Answer from the drawing. Dimensions are ordinates in mm from the lowest x, y and z of the part. A direction names the side the tool comes from. Coordinates: 2 decimals unless noted, no trailing zeros. Order: outer loops, then holes, each group sorted by start corner. A loop starts at its lowest first (then second) coordinate and runs counter-clockwise, first axis right, second up. Notation, with made-up numbers: (-11.75, 27) -> (41.25, 27) arc R24 ccw to (41.25, 47) -> close; hole circle Ø6 at (-15.75, 37.5). An arc over 180 degrees is marked (long way). Answer as a JSON object with one key per item and string values. Group by question number.
1) Section A-A on z = 14.5 is taken. Determine the outline of the cut face in (x, y), and give its area (3 significant figures).
2) Section B-B on x = 20 is taken. Determine the outline of the cut face in (y, z), and give its area (3 significant figures).
3) Determine the mould class of the marked faces 1, 2 and 3 for opening direction X: released by +X, released by -X, zero draft, split by the parting line, or undercut.
4) Section C-C on y = 15 is taken. Determine the outline of the cut face in (x, z), and give its area (3 significant figures).
5) A tool of negligible diameter and unlimited length cuts with its end or side. For the marked faces 4, 5 and 6, from which of +Z, -Z, +X, -X, +Y, -Y can it reach the whole face along a straight path? Write none if from no direction.
6) Consider L1, parallel to Y at x = 20, z = 1.75; L2, parallel to Z at x = 34, y = 13.5; L3, parallel to Z at x = 27.5, y = 32. Determine where each line is inside the solid, lowest interval first.
7) Given pin 1 (12 mm diameter, centred on x = 12, y = 36.5, fed in from +Z); pin 2 (9 mm diameter, centred on x = 34.5, z = 10.5, fed in from +Y), each flat-ended and moving along its own axis, determine where each tip first touches the part or whether it passes through.
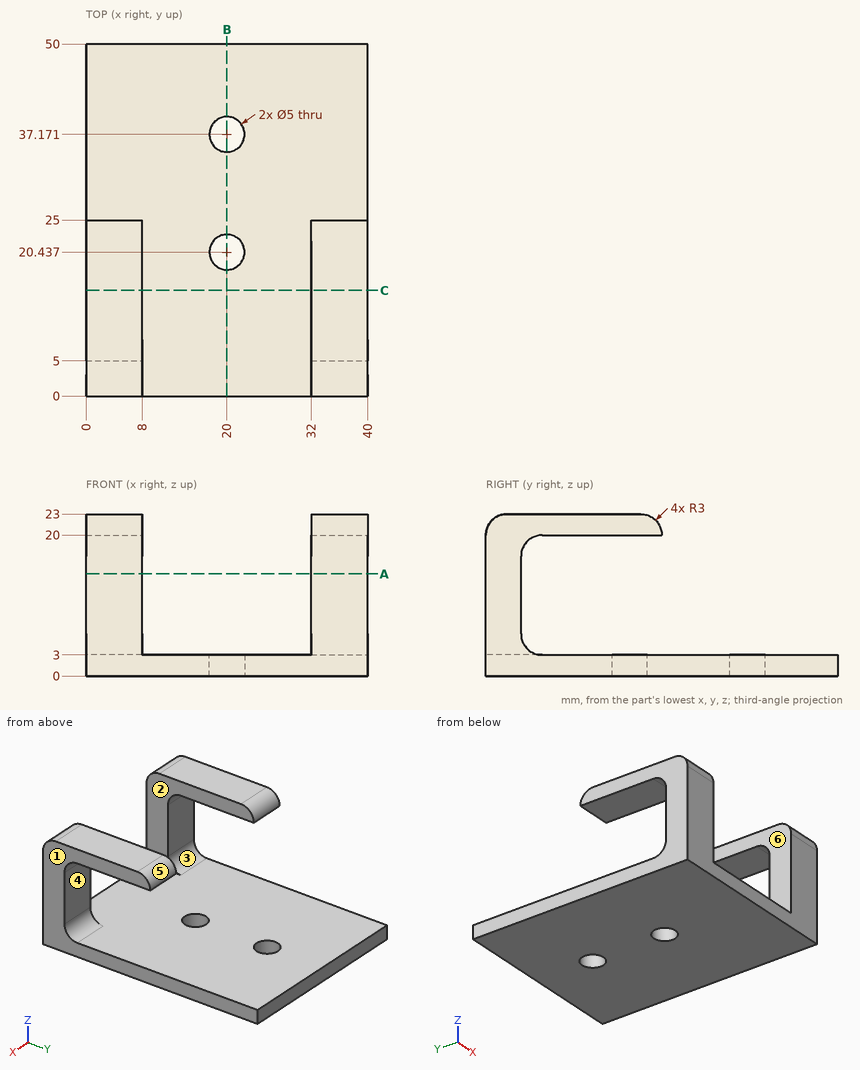
Worked answers:
{
 "1": {"outline": "(0, 0) -> (8, 0) -> (8, 5) -> (0, 5) -> close; (32, 0) -> (40, 0) -> (40, 5) -> (32, 5) -> close", "area": "80.0 mm²"},
 "2": {"outline": "(0, 0) -> (17.94, 0) -> (17.94, 3) -> (0, 3) -> close; (22.94, 0) -> (34.67, 0) -> (34.67, 3) -> (22.94, 3) -> close; (39.67, 0) -> (50, 0) -> (50, 3) -> (39.67, 3) -> close", "area": "120 mm²"},
 "3": {"face 1": "released by +X", "face 2": "undercut", "face 3": "zero draft"},
 "4": {"outline": "(0, 0) -> (40, 0) -> (40, 3) -> (0, 3) -> close; (0, 20) -> (8, 20) -> (8, 23) -> (0, 23) -> close; (32, 20) -> (40, 20) -> (40, 23) -> (32, 23) -> close", "area": "168 mm²"},
 "5": {"face 4": "+X, -X, +Y", "face 5": "+Z, +X, -X, +Y", "face 6": "+Z, +Y, -Y"},
 "6": {"L1": "y = 0 to 17.94, 22.94 to 34.67, 39.67 to 50", "L2": "z = 0 to 3, 20 to 23", "L3": "z = 0 to 3"},
 "7": {"pin 1": "stops at z = 3", "pin 2": "stops at y = 5"}
}
